Could you check a few things on this model? Use its own coordinates, in mm. Face numbers are marked on the shaded views. A direction names the side the tool comes from. Give positions to 0.01 mm unless a question says otherwise; leave off trailing zeros. Write each loop counter-clockwise with the first axis right and the second up, starting at its lowest first coordinate (ties: lowest second). Pieces come first, ordered by that corner, then holes. Notation, with made-up numbers: M 86.5,81.5 L 144.5,81.5 A35 cw 144.5,114.5 Z; hole C -8.5,20.5 d7. An arc over 180 degrees is marked long. One line per item, written item: value.
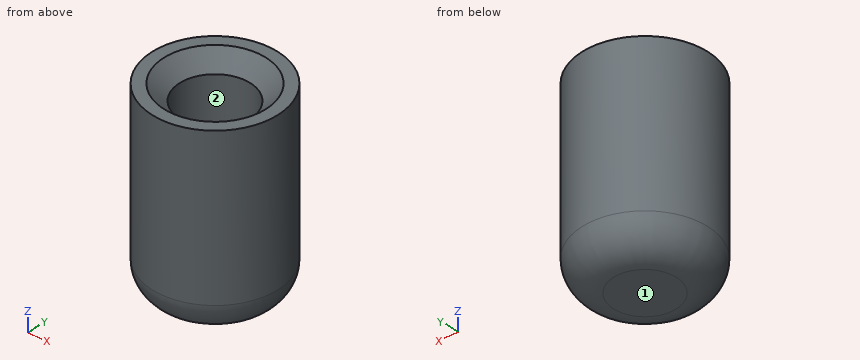
```python
from build123d import *

# Parameters (mm, degrees)
SKETCH_R     = 2
PAD_DEPTH    = 6
SKETCH001_R  = 1.125
POCKET_DEPTH = 5
CHAMFER_SIZE = 0.5
FILLET_R     = 1


with BuildPart() as part:
    # Sketch → Pad (new body)
    with BuildSketch(Plane.XY):
        Circle(SKETCH_R)
    extrude(amount=PAD_DEPTH)

    # Sketch001 (on Face3 of Pad) → Pocket (cut)
    with BuildSketch(Plane.XY.offset(6)):
        Circle(SKETCH001_R)
    extrude(amount=-POCKET_DEPTH, mode=Mode.SUBTRACT)

    # Chamfer
    chamfer_edges = [part.edges().sort_by_distance(p)[0] for p in [
        (-1.125, 0, 6),
    ]]
    chamfer(chamfer_edges, length=CHAMFER_SIZE)

    # Fillet
    fillet_edges = [part.edges().sort_by_distance(p)[0] for p in [
        (-2, 0, 0),
    ]]
    fillet(fillet_edges, radius=FILLET_R)


solid = part.part
```
1) On a 3-axis mill with a long thin cutter (end or side, diameter ignored), from which of +Z, -Z, +X, -X, +Y, -Y can I reach the whole of each face in a straight line? I mean the marked faces 1 and 2. Say none if no direction works.
Outcome:
face 1: -Z, +X, -X, +Y, -Y
face 2: +Z
2) Please list where these lines run through material, in increasing order: L1, parallel to Y at x = 0, z = 2.1 (3 decimals); L2, parallel to Z at x = -0.4, y = 0.7; L3, parallel to X at y = -0.05, z = 1.3. Write a range as from..to.
Outcome:
L1: y = -2..-1.125, 1.125..2
L2: z = 0..1
L3: x = -2..-1.12, 1.12..2
3) I'm going to push flat-ended pins straight in: pin 1 (0.7 mm diameter, centred on x = -0.5, y = -0.5, fed in from +Z); pin 2 (1.5 mm diameter, centred on x = -1, z = 1, fed in from -Y). Where does each tip first touch, or does it pass through?
Outcome:
pin 1: stops at z = 1
pin 2: stops at y = -1.98
4) If we section it at A-A, the plane z = 3.1: Write out the boundary of the cut face in (x, y) (3 decimals), then the cut area to 3 significant figures.
Outcome:
outline: C 0,0 d4; hole C 0,0 d2.25
area: 8.59 mm^2
